Verification items for this drawing (mm, ordinates from the low corner). A direction names the side the tool comes from. Round coordinates to 2 decimals unless told otherwise and drop trailing zeros. Order: outer loops, then holes, each group sorted by start corner. A loop starts at its lowest first (then second) coordinate and runs counter-clockwise, first axis right, second up. Notation, with made-up numbers: (-22.5, -21.5) - (14.5, -21.5) arc R21 cw to (14.5, 6.5) - close; hole circle Ø11 at (80.25, -10.75). An arc over 180 degrees is marked (long way). Use a Markdown table: item, result. Add a question column.
(1) Mould release check, pull along Z, two halves, no side actions. Record for the marked faces 4, 5 and 6: released by +Z, released by -Z, zero draft, split by the parting line, or undercut.
(2) Thickness scan on line 1 along Z through (x, y) = (20, 4.25); line 2 along X through (y, z) = (7, 10); line 3 along X through (y, z) = (13.5, 10). Record the ranges inside material, lowest first. Write a range as [from, to].
(3) Gauge pin test, flat end, axial feed: P1, Ø4.5, axis at x = 19.5, z = 13, coming from the +Y side. Record the tip position at first contact, or that the pin passes through.
(4) Access from +Z, -Z, +X, -X, +Y, -Y to the whole of each face (thin tool, end or side, straight path). Record for the marked faces 1, 2 and 3.
(5) Section check D-D on y = 6.25. Record the boundary of the cut face in (x, z), then the cut area to 3 significant figures.
(6) Section check A-A on y = 15. Record the boundary of the cut face in (x, z).
(7) Section check C-C on x = 20. Record the boundary of the cut face in (y, z).
(8) Section check B-B on z = 10. Record the boundary of the cut face in (x, y), then the cut area to 3 significant figures.
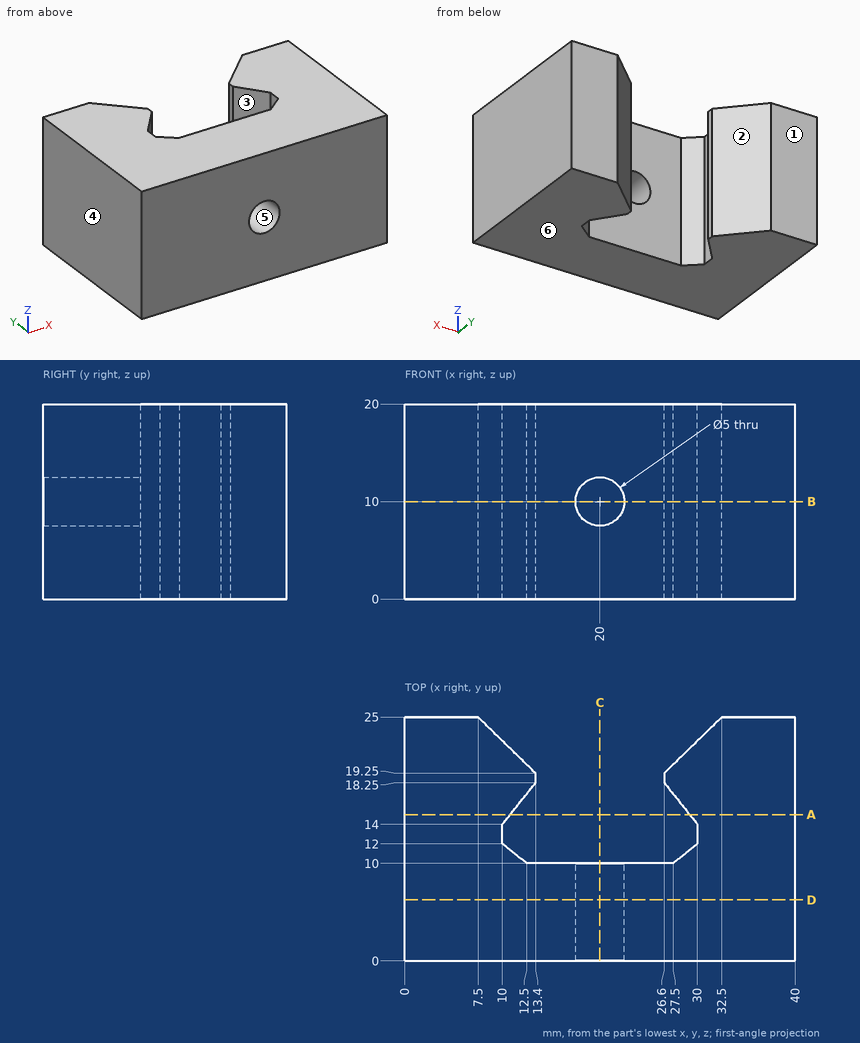
Check sheet entries:
| question | item | result |
|---|---|---|
| 1 | face 4 | zero draft |
| 1 | face 5 | undercut |
| 1 | face 6 | released by -Z |
| 2 | line 1 | z = [0, 7.5], [12.5, 20] |
| 2 | line 2 | x = [0, 17.5], [22.5, 40] |
| 2 | line 3 | x = [0, 10], [30, 40] |
| 3 | P1 | stops at y = 10 |
| 4 | face 1 | +Z, -Z, +X, -X, +Y |
| 4 | face 2 | +Z, -Z, +Y |
| 4 | face 3 | +Z, -Z |
| 5 | outline | (0, 0) - (40, 0) - (40, 20) - (0, 20) - close; hole circle Ø5 at (20, 10) |
| 5 | area | 780 mm2 |
| 6 | outline | (0, 0) - (10.8, 0) - (10.8, 20) - (0, 20) - close; (29.2, 0) - (40, 0) - (40, 20) - (29.2, 20) - close |
| 7 | outline | (0, 0) - (10, 0) - (10, 7.5) - (0, 7.5) - close; (0, 12.5) - (10, 12.5) - (10, 20) - (0, 20) - close |
| 8 | outline | (0, 0) - (17.5, 0) - (17.5, 10) - (12.5, 10) - (10, 12) - (10, 14) - (13.4, 18.25) - (13.4, 19.25) - (7.5, 25) - (0, 25) - close; (22.5, 0) - (40, 0) - (40, 25) - (32.5, 25) - (26.6, 19.25) - (26.6, 18.25) - (30, 14) - (30, 12) - (27.5, 10) - (22.5, 10) - close |
| 8 | area | 681 mm2 |
